Design review of the part built by this model. Coordinates are the model's own, in mm. A direction names the side the tool comes from. Give positions to 0.01 mm unless a question says otherwise; leave off trailing zeros. Loops run counter-clockwise (first coordinate to the right, second up) from the corner with the lowest first, then second, coordinate; pieces in that order, holes last. Notation, with made-up numbers: (-1.5, 41.5) -> (53.5, 41.5) arc R20 ccw to (53.5, 74.5) -> close; hole circle Ø7 at (-21.75, -9). An arc over 180 degrees is marked (long way). Use a Markdown table: item, result. Add a question column.
1. Add section B-B (z = 4.75). Count the separate pieces of the cut face and the enclosed holes in it, and give its area (3 significant figures).
2. To check wall thickness, follow line 1 (Y direction, x = 21.92, z = 6.25) (3 decimals); line 2 (X direction, y = -19.5, z = 6.5); line 3 (Y direction, x = -10, z = 5.15). State the ranges of each line that lie inside material, in increasing order.
3. For pin 1 Ø4 at (x, z) = (-18, 6) entering from -Y; pin 2 Ø2 at (x, y) = (-9.5, -18) entering from +Z; pin 3 Ø2 at (x, z) = (-19, 3.5) entering from -Y, all flat-tipped, find the tip position at first contact; note any pin that passes through.
4. Add section A-A (y = -18.1). State the section outline as (x, z) points (3 decimals).
5. For faces 1 (the cylindrical face through (-0.288, -0.102, 3.944)), 2 (the flat face through (10, -18, 4)), list the 3-axis set-ups (+Z, -Z, +X, -X, +Y, -Y) from which the entire face can be reached by the end or side of a thin tool; tool diameter is ignored.
6. Draft analysis for pull direction X (two halves, no side actions). For faces 3 (the cylindrical face through (-22.97, -17.29, 3.94)), 4 (the cylindrical face through (0.288, -36.098, 3.944)), 5 (the flat face through (0, -18, 8)), state which applies: pulls with the +X half, pulls with the -X half, needs draft (parallel to the pull), parting line crosses it, or undercut.
7. Add section C-C (x = -10). State the section outline as (y, z) points.
Autodesk Inventor part; units mm, degrees
ref_plane "YZ Plane" through (0, 0, 0) normal (1, 0, 0) x (0, 1, 0)
ref_plane "XZ Plane" through (0, 0, 0) normal (0, 1, 0) x (-1, 0, 0)
ref_plane "XY Plane" through (0, 0, 0) normal (0, 0, 1) x (1, 0, 0)
sketch "Sketch1" plane through (0, 0, 0) normal (0, 0, 1) x (1, 0, 0)
  circle A0 centre (0, -18.1) radius 17.9
  circle A1 centre (0, -18.1) radius 2.9
  circle A2 centre (-13.5, -18.1) radius 1.525
  circle A3 centre (13.5, -18.1) radius 1.525
  circle A4 centre (0, -18.1) radius 18
  arc A5 (23.0705, -21.2782) -> (23.0705, -14.9218) centre (21.92, -18.1) ccw
  line L0 (23.0705, -14.9218) -> (17.5529, -12.9245)
  arc A6 (17.5529, -23.2755) -> (17.5529, -12.9245) centre (0, -18.1) ccw
  line L1 (17.5529, -23.2755) -> (23.0705, -21.2782)
  circle A7 centre (21.92, -18.1) radius 1.325
  arc A8 (-23.0705, -14.9218) -> (-23.0705, -21.2782) centre (-21.92, -18.1) ccw
  line L2 (-23.0705, -21.2782) -> (-17.5529, -23.2755)
  arc A9 (-17.5529, -12.9245) -> (-17.5529, -23.2755) centre (0, -18.1) ccw
  line L3 (-17.5529, -12.9245) -> (-23.0705, -14.9218)
  circle A10 centre (-21.92, -18.1) radius 1.325
  line L4 (0, -18.1) -> (-21.92, -18.1)
  line L5 (-21.92, -18.1) -> (21.92, -18.1)
  circle A11 centre (21.92, -18.1) radius 4
  circle A12 centre (-21.92, -18.1) radius 4
  circle A13 centre (21.8177, -28.0995) radius 6
  circle A14 centre (21.8177, -8.1005) radius 6
  circle A15 centre (-21.8177, -28.0995) radius 6
  circle A16 centre (-21.8177, -8.1005) radius 6
  point P0 (0, 0)
  point P1 (16.3632, -25.5996)
  point P2 (21.8791, -22.0998)
  point P3 (21.8791, -14.1002)
  point P4 (16.3632, -10.6004)
  point P5 (-16.3632, -10.6004)
  point P6 (-21.8791, -14.1002)
  point P7 (-21.8791, -22.0998)
  point P8 (-16.3632, -25.5996)
  dimension "d0" = 36
  dimension "d1" = 8
  dimension "d2" = 8
  dimension "d3" = 12
  dimension "d4" = 12
  dimension "d5" = 12
  dimension "d6" = 12
extrude "Extrusion1" add sketch "Sketch1" along normal blind 8 contours L5 A3 A1 L4 A2 A0 | L5 A11 A4 A12 L4 A0 | A0 L4 A2 A1 L5 A3 | A0 L4 A12 A4 A11 L5 | L5 A3 | A3 L5 | A11 A4 L5 | L5 A4 A11 | L4 A2 | A2 L4 | A12 A4 L4 | L4 A4 A12 | L5 A6 A11 A4 | A4 A11 A6 L5 | A4 A14 L0 A6 A11 | A11 A6 L1 A13 A4 | L4 A9 A12 A4 | A4 A12 A9 L4 | A12 A9 L3 A16 A4 | A4 A15 L2 A9 A12 | L5 L4 A1 | A1 L4 L5 | A6 A11 L0 A5 L1 | A6 L0 A14 A11 | A11 L1 A13 A6 | A9 A12 L2 A8 L3 | A12 L3 A16 A9 | A9 L2 A15 A12 | A11 L1 A5 L0 | L0 A14 A11 | A11 A13 L1 | A12 A16 L3 | L3 A8 L2 A12 | L2 A15 A12
sketch "Sketch2" plane through (0, 0, 8) normal (0, 0, 1) x (1, 0, 0)
  circle A0 centre (21.92, -18.1) radius 1.325
  circle A1 centre (-21.92, -18.1) radius 1.325
  line L0 (21.92, -18.1) -> (-21.92, -18.1)
  line L1 (0, -18.1) -> (-10, -18.1)
  line L2 (0, -18.1) -> (10, -18.1)
  point P0 (0, 0)
  dimension "d9" = 10
  dimension "d10" = 10
hole "Hole1" at (10, -18.1, 8) at (-10, -18.1, 8) direction (0, 0, -1) diameter 4.134 depth 4
properties part number "extruder waterblock"
Taken from the geometry:
| question | item | result |
|---|---|---|
| 1 | separate pieces | 1 |
| 1 | enclosed holes | 4 |
| 1 | area | 1,110 mm^2 |
| 2 | line 1 | y = -22.1 to -19.425, -16.775 to -14.1 |
| 2 | line 2 | x = -25.67 to -11.52, -8.48 to 8.48, 11.52 to 25.67 |
| 2 | line 3 | y = -33.07 to -20.17, -16.03 to -3.13 |
| 3 | pin 1 | stops at y = -26.35 |
| 3 | pin 2 | stops at z = 4 |
| 3 | pin 3 | stops at y = -23.47 |
| 4 | outline | (-25.92, 0) -> (-23.245, 0) -> (-23.245, 8) -> (-25.92, 8) -> close; (-20.595, 0) -> (20.595, 0) -> (20.595, 8) -> (12.067, 8) -> (12.067, 4) -> (7.933, 4) -> (7.933, 8) -> (-7.933, 8) -> (-7.933, 4) -> (-12.067, 4) -> (-12.067, 8) -> (-20.595, 8) -> close; (23.245, 0) -> (25.92, 0) -> (25.92, 8) -> (23.245, 8) -> close |
| 5 | face 1 | +Z, -Z, +Y |
| 5 | face 2 | +Z |
| 6 | face 3 | undercut |
| 6 | face 4 | parting line crosses it |
| 6 | face 5 | needs draft |
| 7 | outline | (-33.07, 0) -> (-3.13, 0) -> (-3.13, 8) -> (-16.03, 8) -> (-16.03, 4) -> (-20.17, 4) -> (-20.17, 8) -> (-33.07, 8) -> close |
